from build123d import *

# Parameters (mm, degrees)
F0_W     = 101.6
F0_H     = 107.734338
F0_R     = 24.735745
F2_DEPTH = 76.2
F1_R     = 30.273775
F3_DEPTH = 101.6
F5_D     = 50.8


with BuildPart() as f2:
    # F0 (on Front) → F2 (new body)
    with BuildSketch(Plane.XZ):
        with Locations((0, 1.91698)):
            Rectangle(F0_W, F0_H)
        Circle(F0_R, mode=Mode.SUBTRACT)
    extrude(amount=F2_DEPTH)

    # F1 (on Front) → F3 (join)
    with BuildSketch(Plane.XZ):
        Circle(F1_R)
    extrude(amount=F3_DEPTH)

    # F5 (through all)
    with Locations(Plane(origin=(0, 0, 0), x_dir=(1, 0, 0), z_dir=(0, 1, 0))):
        with Locations((0, 0)):
            Hole(F5_D / 2)


solid = f2.part
Input: part model. Units: mm. Frame: model coordinates. A direction names the side the tool comes from. Round coordinates to 2 decimals unless told otherwise and drop trailing zeros. Write each loop counter-clockwise with the first axis right and the second up, starting at its lowest first coordinate (ties: lowest second). Pieces come first, ordered by that corner, then holes.
1) Reachability of faces 5 (the flat face through (-1, -38, 55.784)), 6 (the flat face through (22, -76.2, 27)) from +Z, -Z, +X, -X, +Y, -Y: full face, straight path, thin tool, end or side. Return the list, or none.
2) Contact query for a flat-ended pin moving along its axis: P1, Ø10, axis at x = 23.5, z = 31.5, coming from the -Y side. Output: stop coordinate, or through.
3) Cut plane B-B (x = 0). Return the cut outline in (y, z).
4) Cut plane C-C (y = -23). Return the cut outline in (x, z), then the cut area to 3 significant figures.
5) Cut plane D-D (x = 45.5). Return the cut outline in (y, z).
6) Ray query, L1, parallel to Z at x = 0, y = -80; L2, parallel to Z at x = 0, y = -58; L3, parallel to Y at x = 46, z = 3. Return the intervals inside material, ascending.
7) Cut plane A-A (z = 0). Return the cut outline in (x, y), then the cut area to 3 significant figures.
8) Draft query along Z for faces 1 (the flat face through (-1, -38, -51.95)), 2 (the cylindrical face through (5.506, -51.511, 24.796)), 3 (the cylindrical face through (-3.941, -88.722, 30.016)), 4 (the flat face through (-1, 0, 27)). Return one class per face: pulls with the +Z half, pulls with the -Z half, needs draft (parallel to the pull), parting line crosses it, or undercut.
Geometry says:
1. face 5: +Z, +X, -X, +Y, -Y
1. face 6: -Y
2. P1: stops at y = -76.2
3. outline: (-101.6, -30.27) - (-76.2, -30.27) - (-76.2, -51.95) - (0, -51.95) - (0, -25.4) - (-101.6, -25.4) - close; (-101.6, 25.4) - (0, 25.4) - (0, 55.78) - (-76.2, 55.78) - (-76.2, 30.27) - (-101.6, 30.27) - close
4. outline: (-50.8, -51.95) - (50.8, -51.95) - (50.8, 55.78) - (-50.8, 55.78) - close; hole circle Ø50.8 at (0, 0)
4. area: 8,920 mm2
5. outline: (-76.2, -51.95) - (0, -51.95) - (0, 55.78) - (-76.2, 55.78) - close
6. L1: z = -30.27 to -25.4, 25.4 to 30.27
6. L2: z = -51.95 to -25.4, 25.4 to 55.78
6. L3: y = -76.2 to 0
7. outline: (-50.8, -76.2) - (-30.27, -76.2) - (-30.27, -101.6) - (-25.4, -101.6) - (-25.4, 0) - (-50.8, 0) - close; (25.4, -101.6) - (30.27, -101.6) - (30.27, -76.2) - (50.8, -76.2) - (50.8, 0) - (25.4, 0) - close
7. area: 4,120 mm2
8. face 1: pulls with the -Z half
8. face 2: undercut
8. face 3: parting line crosses it
8. face 4: needs draft
